The drawing under review shows one solid part. Ordinate dimensions are in mm from its lowest x, y, z. A direction names the side the tool comes from. Round coordinates to 2 decimals unless told otherwise and drop trailing zeros. Order: outer loops, then holes, each group sorted by start corner. A loop starts at its lowest first (then second) coordinate and runs counter-clockwise, first axis right, second up. Notation, with made-up numbers: (-15, 87.25) - (-3, 87.25) arc R19 ccw to (-3, 116.25) - close; hole circle Ø7 at (-3, -11.5). An arc over 180 degrees is marked (long way). Answer as a JSON object with one key per item and string values. Group by question number.
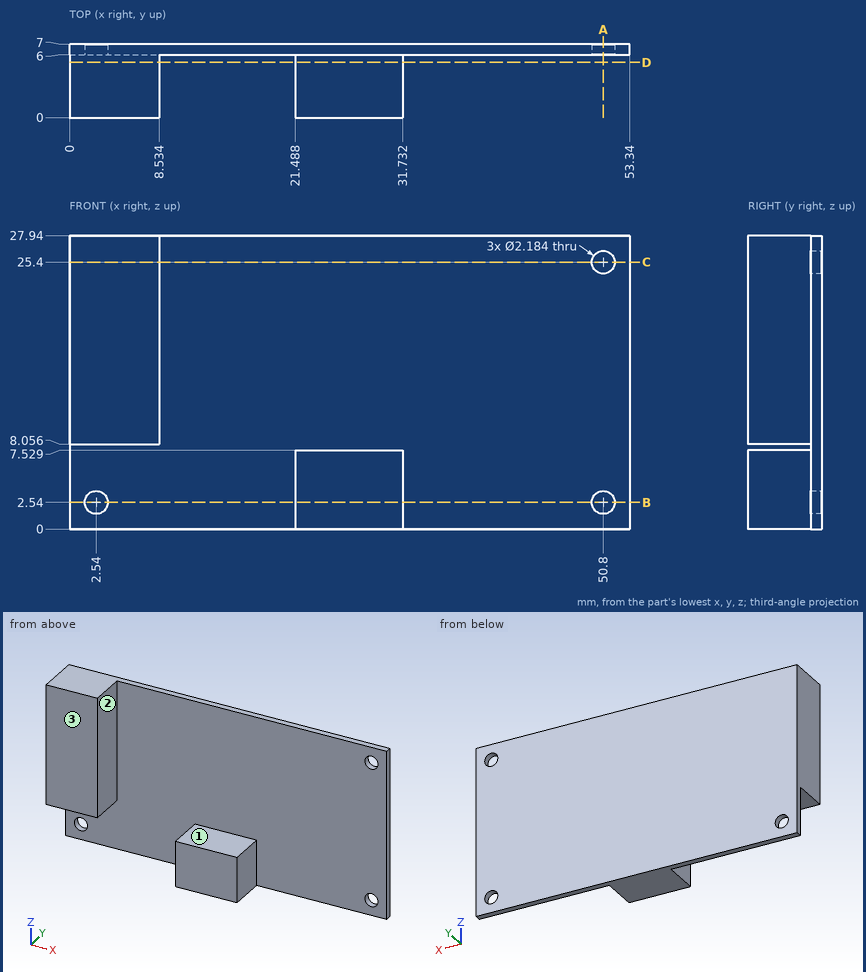
1. To check wall thickness, follow line 1 (X direction, y = 6.8, z = 25.4); line 2 (Y direction, x = 30, z = 13.5); line 3 (X direction, y = 5.25, z = 16). State the ranges of each line that lie inside material, in increasing order. Write a range as from..to.
2. Clearance check with flat-ended pins moving along their axes: P1, Ø12, axis at x = 44.5, z = 24.5, coming from the -Y side; P2, Ø1.7, axis at x = 50.8, z = 25.4, coming from the +Y side; P3, Ø3, axis at y = 2, z = 17, coming from the +X side; P4, Ø1.8, axis at y = 4, z = 3, coming from the -X side. State where each tip first meets the part, or that it passes through.
3. Take a section at A-A, the plane x = 50.8. Give the boundary of the cut face in (y, z).
4. Take a section at C-C, the plane z = 25.4. Give the boundary of the cut face in (x, y), then the cut area to 3 significant figures.
5. Take a section at B-B, the plane z = 2.54. Give the boundary of the cut face in (x, y).
6. Tool access review of the marked faces 1, 2 and 3: name each direction out of +Z, -Z, +X, -X, +Y, -Y from which nothing blocks a thin tool from reaching the whole face with its end or side.
7. Take a section at D-D, the plane y = 5.25. Give the boundary of the cut face in (x, z), then the cut area to 3 significant figures.
Response values:
{
 "1": {"line 1": "0..49.71, 51.89..53.34", "line 2": "6..7", "line 3": "0..8.53"},
 "2": {"P1": "y = 6", "P2": "through", "P3": "x = 8.53", "P4": "x = 21.49"},
 "3": {"outline": "(6, 0) - (7, 0) - (7, 1.45) - (6, 1.45) - close; (6, 3.63) - (7, 3.63) - (7, 24.31) - (6, 24.31) - close; (6, 26.49) - (7, 26.49) - (7, 27.94) - (6, 27.94) - close"},
 "4": {"outline": "(0, 0) - (8.53, 0) - (8.53, 6) - (49.71, 6) - (49.71, 7) - (0, 7) - close; (51.89, 6) - (53.34, 6) - (53.34, 7) - (51.89, 7) - close", "area": "102 mm2"},
 "5": {"outline": "(0, 6) - (1.45, 6) - (1.45, 7) - (0, 7) - close; (3.63, 6) - (21.49, 6) - (21.49, 0) - (31.73, 0) - (31.73, 6) - (49.71, 6) - (49.71, 7) - (3.63, 7) - close; (51.89, 6) - (53.34, 6) - (53.34, 7) - (51.89, 7) - close"},
 "6": {"face 1": "+Z, +X, -X, -Y", "face 2": "+Z, -Z, +X, -Y", "face 3": "+Z, -Z, +X, -X, -Y"},
 "7": {"outline": "(0, 8.06) - (8.53, 8.06) - (8.53, 27.94) - (0, 27.94) - close; (21.49, 0) - (31.73, 0) - (31.73, 7.53) - (21.49, 7.53) - close", "area": "247 mm2"}
}
